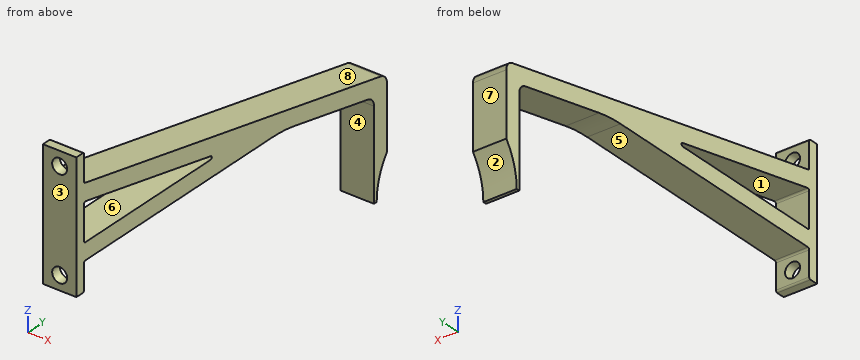
from build123d import *

# Parameters (mm, degrees)
BOSS_EXTRUDE1_DEPTH = 10
SKETCH1_5_OUTSIDE_W = 96.286
SKETCH1_5_OUTSIDE_H = 149.536
CUT_EXTRUDE2_DEPTH  = 10
SKETCH5_R           = 2.25
CUT_EXTRUDE3_DEPTH  = 10


with BuildPart() as part:
    # Sketch1 → Boss-Extrude1 (new body)
    with BuildSketch(Plane(origin=(0, 0, 0), x_dir=(0, 0, -1), z_dir=(1, 0, 0))):
        with BuildLine():
            Line((19.39483456, 104.718712665), (-4.885010669, -9.508978253))
            ThreePointArc((-4.885010669, -9.508978253), (-5.059424274, -9.793595388), (-5.374084469, -9.905022408))
            Line((-5.374084469, -9.905022408), (-12.969192453, -9.905022408))
            ThreePointArc((-12.969192453, -9.905022408), (-13.322745843, -10.051469017), (-13.469192453, -10.405022408))
            Line((-13.469192453, -10.405022408), (-13.469192453, -12.905022408))
            Line((-13.469192453, -12.905022408), (25.030807547, -12.905022408))
            Line((25.030807547, -12.905022408), (25.030807547, -10.405022408))
            ThreePointArc((25.030807547, -10.405022408), (24.884360938, -10.051469017), (24.530807547, -9.905022408))
            Line((24.530807547, -9.905022408), (17.030807547, -9.905022408))
            ThreePointArc((17.030807547, -9.905022408), (16.677254157, -9.758575798), (16.530807547, -9.405022408))
            Line((16.530807547, -9.405022408), (16.530807547, 62.991683812))
            ThreePointArc((16.530807547, 62.991683812), (16.749931733, 67.172822342), (17.404903518, 71.308151444))
            Line((17.404903518, 71.308151444), (23.443754726, 99.718712665))
            ThreePointArc((23.443754726, 99.718712665), (24.490236355, 101.426415477), (26.378197528, 102.094977592))
            Line((26.378197528, 102.094977592), (53.280807547, 102.094977592))
            Line((53.280807547, 102.094977592), (53.280807547, 103.094977592))
            ThreePointArc((53.280807547, 103.094977592), (46.956252227, 104.121311631), (41.280807547, 107.094977592))
            Line((41.280807547, 107.094977592), (22.329277362, 107.094977592))
            ThreePointArc((22.329277362, 107.094977592), (20.441316189, 106.426415477), (19.39483456, 104.718712665))
        make_face()
    extrude(amount=BOSS_EXTRUDE1_DEPTH)

    # Sketch1_5 outside → Cut-Extrude2 (cut)
    # profile 1 of 2: a face of its own
    with BuildSketch(Plane(origin=(0, 0, 0), x_dir=(0, 0, -1), z_dir=(1, 0, 0))):
        with Locations((19.906, 47.095)):
            Rectangle(SKETCH1_5_OUTSIDE_W, SKETCH1_5_OUTSIDE_H)
        with BuildLine():
            Line((19.39483456, 104.718712665), (-4.885010669, -9.508978253))
            ThreePointArc((-4.885010669, -9.508978253), (-5.059424274, -9.793595388), (-5.374084469, -9.905022408))
            Line((-5.374084469, -9.905022408), (-12.969192453, -9.905022408))
            ThreePointArc((-12.969192453, -9.905022408), (-13.322745843, -10.051469017), (-13.469192453, -10.405022408))
            Line((-13.469192453, -10.405022408), (-13.469192453, -12.905022408))
            Line((-13.469192453, -12.905022408), (25.030807547, -12.905022408))
            Line((25.030807547, -12.905022408), (25.030807547, -10.405022408))
            ThreePointArc((25.030807547, -10.405022408), (24.884360938, -10.051469017), (24.530807547, -9.905022408))
            Line((24.530807547, -9.905022408), (17.030807547, -9.905022408))
            ThreePointArc((17.030807547, -9.905022408), (16.677254157, -9.758575798), (16.530807547, -9.405022408))
            Line((16.530807547, -9.405022408), (16.530807547, 62.991683812))
            ThreePointArc((16.530807547, 62.991683812), (16.749931733, 67.172822342), (17.404903518, 71.308151444))
            Line((17.404903518, 71.308151444), (23.443754726, 99.718712665))
            ThreePointArc((23.443754726, 99.718712665), (24.490236355, 101.426415477), (26.378197528, 102.094977592))
            Line((26.378197528, 102.094977592), (53.280807547, 102.094977592))
            Line((53.280807547, 102.094977592), (53.280807547, 103.094977592))
            ThreePointArc((53.280807547, 103.094977592), (46.956252227, 104.121311631), (41.280807547, 107.094977592))
            Line((41.280807547, 107.094977592), (22.329277362, 107.094977592))
            ThreePointArc((22.329277362, 107.094977592), (20.441316189, 106.426415477), (19.39483456, 104.718712665))
        make_face(mode=Mode.SUBTRACT)
    # profile 2 of 2: a face of its own
    with BuildSketch(Plane(origin=(0, 0, 0), x_dir=(0, 0, -1), z_dir=(1, 0, 0))):
        with BuildLine():
            Line((0.7599591, -9.905022408), (11.030807547, -9.905022408))
            ThreePointArc((11.030807547, -9.905022408), (11.384360938, -9.758575798), (11.530807547, -9.405022408))
            Line((11.530807547, -9.405022408), (11.530807547, 38.915520448))
            ThreePointArc((11.530807547, 38.915520448), (11.083071779, 39.412781396), (10.541733747, 39.019476293))
            Line((10.541733747, 39.019476293), (0.2708853, -9.301066562))
            ThreePointArc((0.2708853, -9.301066562), (0.371386119, -9.719682603), (0.7599591, -9.905022408))
        make_face()
    extrude(amount=CUT_EXTRUDE2_DEPTH, mode=Mode.SUBTRACT)

    # Sketch5 → Cut-Extrude3 (cut)
    with BuildSketch(Plane.XZ.offset(12.905022408)):
        with Locations(Location((5, 9.219192453, 0), (0, 0, 270))):
            Circle(SKETCH5_R)
        with Locations(Location((5, -20.780807547, 0), (0, 0, 270))):
            Circle(SKETCH5_R)
    extrude(amount=-CUT_EXTRUDE3_DEPTH, mode=Mode.SUBTRACT)


solid = part.part
Here's how the part is built. I have some questions about the finished solid (model axes, mm). Face numbers are marked on the shaded views. A direction names the side the tool comes from. Round coordinates to 2 decimals unless told otherwise and drop trailing zeros. Order: outer loops, then holes, each group sorted by start corner. A loop starts at its lowest first (then second) coordinate and runs counter-clockwise, first axis right, second up. Notation, with made-up numbers: (-30, 72) -> (-26, 72) arc R27 cw to (-26, 107) -> close; hole circle Ø7 at (68, 29.25). An arc over 180 degrees is marked (long way). Return JSON: item names as keys, results as strings.
Q1. For pin 1 Ø3 at (x, z) = (3, -46.5) entering from -Y (3 decimals); pin 2 Ø1.2 at (x, y) = (4.5, -12) entering from -Z; pin 3 Ø1.5 at (x, y) = (2.5, 1) entering from +Z, each with a flat end and sliding along its axis, tell me the tip position at first contact or that it passes through.
Filled sheet:
{"pin 1": "stops at y = 102.095", "pin 2": "stops at z = -25.03", "pin 3": "stops at z = 2.81"}
Q2. If we section it at A-A on x = 5: Give the number of separate pieces and of enclosed holes in the cut face, plus the area to 3 significant figures.
Filled sheet:
{"separate pieces": "3", "enclosed holes": "1", "area": "1,130 mm^2"}
Q3. If we section it at B-B on y = 7: List the corners of the cut face in (x, z) for me.
Filled sheet:
{"outline": "(0, -16.53) -> (10, -16.53) -> (10, -11.53) -> (0, -11.53) -> close; (0, -3.74) -> (10, -3.74) -> (10, 1.38) -> (0, 1.38) -> close"}
Q4. If we section it at C-C on z = -7: List the corners of the cut face in (x, y) for me.
Filled sheet:
{"outline": "(0, -12.91) -> (10, -12.91) -> (10, -9.91) -> (0, -9.91) -> close; (0, 22.36) -> (10, 22.36) -> (10, 46.41) -> (0, 46.41) -> close"}
Q5. Which directions (+Z, -Z, +X, -X, +Y, -Y) give clear straight access to the entire face, cutting with the end or side of a thin tool? Please do the marked faces 4, 5, 6, 7 and 8.
Filled sheet:
{"face 4": "-Z, +X, -X, -Y", "face 5": "-Z, +X, -X", "face 6": "+X, -X", "face 7": "+Z, -Z, +X, -X, +Y", "face 8": "+Z, +X, -X, +Y"}
Q6. If we mould it in two halves opening along Z, with no side actions, what happens to the marked faces 1, 2 and 3? For each: released by +Z, released by -Z, zero draft, split by the parting line, or undercut.
Filled sheet:
{"face 1": "undercut", "face 2": "released by -Z", "face 3": "zero draft"}
Q7. If we section it at D-D on z = -48: List the corners of the cut face in (x, y) for me.
Filled sheet:
{"outline": "(0, 102.09) -> (10, 102.09) -> (10, 103.8) -> (0, 103.8) -> close"}
Q8. I need wall thicknesses on line 1 along Y through (x, z) = (6.5, 6.5); line 2 along Z through (x, y) = (7.5, 11); line 3 along Z through (x, y) = (8.5, 58.5). Which ranges of each line are inside material? Lowest first, please. Write a range as from..to.
Filled sheet:
{"line 1": "y = -12.91..-9.91", "line 2": "z = -16.53..-11.53, -4.59..0.53", "line 3": "z = -16.53..-9.57"}
